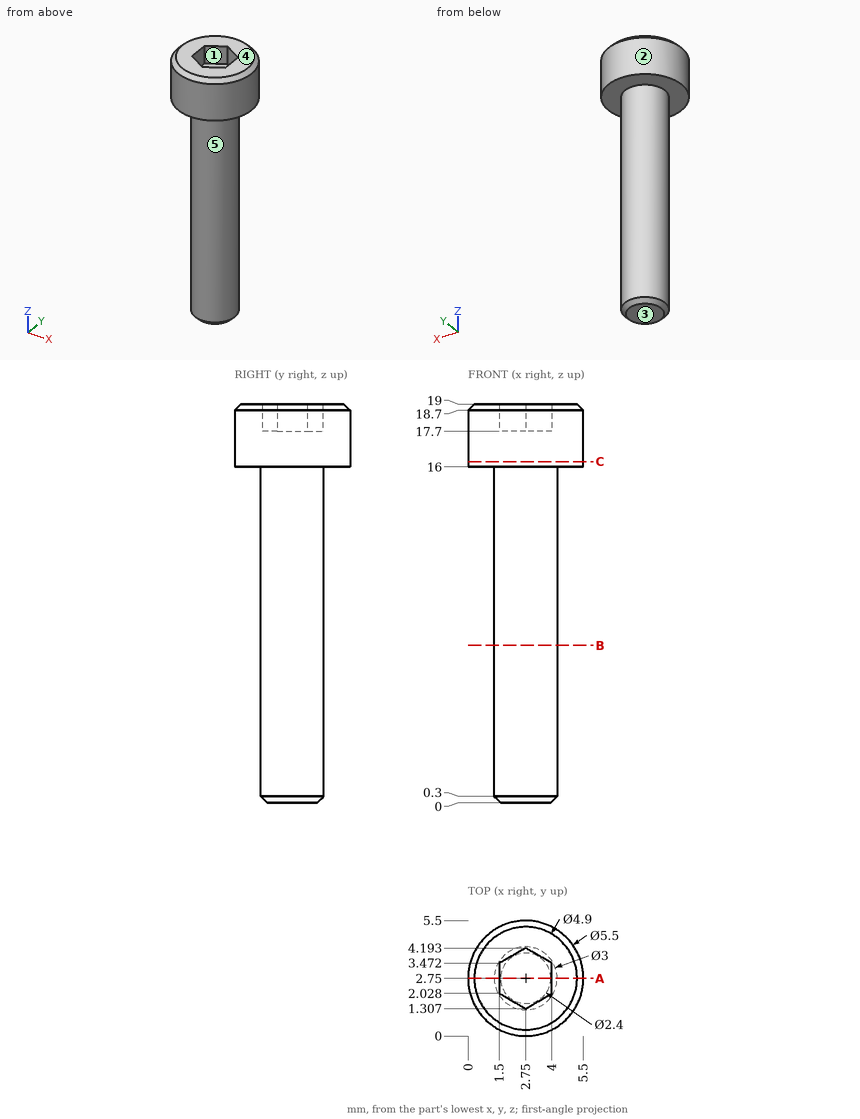
Drawing for the job (mm, zero at the part's lowest x, y, z). A direction names the side the tool comes from. Give positions to 0.01 mm unless a question says otherwise; leave off trailing zeros. Order: outer loops, then holes, each group sorted by start corner. A loop starts at its lowest first (then second) coordinate and runs counter-clockwise, first axis right, second up. Notation, with made-up numbers: M 25,-34.75 L 48,-34.75 A32 cw 48,-4.75 Z; hole C -3.75,86 d5. An arc over 180 degrees is marked long. Use a Markdown table: item, result. Add a question column.
(1) 3-axis set-ups, long thin cutter, end or side, ignore diameter. For the marked faces 4 and 5: which of +Z, -Z, +X, -X, +Y, -Y reach the whole face in a straight line?
(2) Drop flat-ended pins along their axis: P1, Ø3, axis at y = 3.5, z = 3.5, coming from the +X side; P2, Ø1.4, axis at y = 2.5, z = 18.5, coming from the +X side; P3, Ø1.5, axis at x = 3, z = 9.5, coming from the -Y side; P4, Ø1, axis at x = 1, y = 3.5, coming from the -Z side (1 decimal). Give the stop position or say it passes through.
(3) Saw through at C-C, the plane z = 16.25. Give the cut face in (x, y).
(4) Saw through at B-B, the plane z = 7.5. Give the cut face in (x, y).
(5) Mould opens along Y. For the marked faces 1, 2 and 3 say: +Y half, -Y half, draft (parallel to the pull), parting line (faces both ways), or undercut.
(6) Probe line 1 along Z through (x, y) = (4.9, 2.05); line 2 along Z through (x, y) = (2.6, 1.75); line 3 along Y through (x, z) = (2.8, 13.75). List the from-to ranges inside material, lowest first. Write a range as [from, to].
(7) Saw through at A-A, the plane y = 2.75. Give the cut face in (x, z).
Answer key:
| question | item | result |
|---|---|---|
| 1 | face 4 | +Z, +X, -X, +Y, -Y |
| 1 | face 5 | -Z |
| 2 | P1 | x = 4.25 |
| 2 | P2 | x = 5.5 |
| 2 | P3 | y = 1.25 |
| 2 | P4 | z = 0.2 |
| 3 | outline | C 2.75,2.75 d5.5 |
| 4 | outline | C 2.75,2.75 d3 |
| 5 | face 1 | undercut |
| 5 | face 2 | parting line |
| 5 | face 3 | draft |
| 6 | line 1 | [16, 19] |
| 6 | line 2 | [0, 17.7] |
| 6 | line 3 | [1.25, 4.25] |
| 7 | outline | M 0,16 L 1.25,16 L 1.25,0.3 L 1.55,0 L 3.95,0 L 4.25,0.3 L 4.25,16 L 5.5,16 L 5.5,18.7 L 5.2,19 L 4,19 L 4,17.7 L 1.5,17.7 L 1.5,19 L 0.3,19 L 0,18.7 Z |
